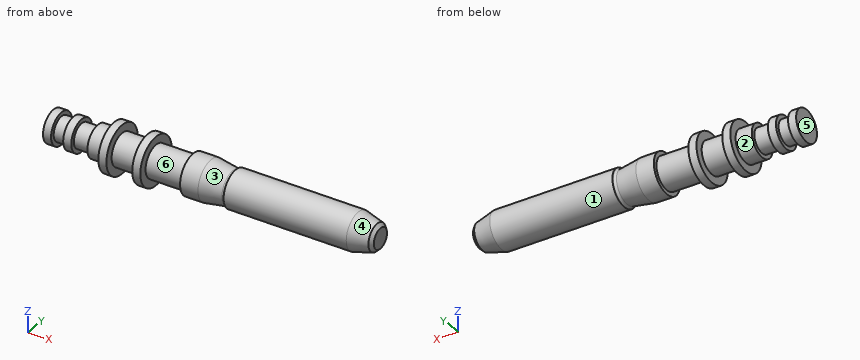
from build123d import *

# Parameters (mm, degrees)
FILLET1_R      = 0.0762
CHAMFER1_SIZE  = 0.0762
CHAMFER1_SIZE2 = 0.107763073


with BuildPart() as part:
    # Sketch1 → Revolve1 (revolve)
    with BuildSketch(Plane.XY, mode=Mode.PRIVATE) as revolve1_sk:
        Polygon((6.955835037, 0.508), (6.955835037, 0), (17.242835037, 0), (17.242835037, 0.397037489), (16.544335037, 0.5842), (12.686075037, 0.5842), (12.648252987, 0.518690288), (11.913915037, 0.635), (11.350035037, 0.635), (11.350035037, 0.508), (10.181635037, 0.508), (10.181635037, 0.762), (9.927635037, 0.762), (9.927635037, 0.508), (9.114835037, 0.508), (9.114835037, 0.762), (8.860835037, 0.762), (8.860835037, 0.508), (8.352835037, 0.508), (8.352835037, 0.381), (7.844835037, 0.381), (7.844835037, 0.508), (7.590835037, 0.508), (7.590835037, 0.381), (7.209835037, 0.381), (7.209835037, 0.508), align=None)
    revolve(revolve1_sk.sketch.rotate(Axis((-986.284560053, 0, 0), (1, 0, 0)), 180), axis=Axis((-986.284560053, 0, 0), (1, 0, 0)))

    # Fillet1
    fillet1_edges = [part.edges().sort_by_distance(p)[0] for p in [
        (12.648252987, 0.518690288, 0),
    ]]
    fillet(fillet1_edges, radius=FILLET1_R)

    # Chamfer1
    chamfer1_edges = [part.edges().sort_by_distance(p)[0] for p in [
        (17.242835037, 0.397037489, 0),
    ]]
    chamfer1_side = [part.faces().sort_by_distance(p)[0] for p in [
        (17.242835037, 0, 0),
    ]]
    chamfer(chamfer1_edges, length=CHAMFER1_SIZE, length2=CHAMFER1_SIZE2, reference=chamfer1_side[0])


solid = part.part
Work out the finished part from the listing and answer in its coordinate system (mm). Face numbers are marked on the shaded views. A direction names the side the tool comes from. Coordinates: 2 decimals unless noted, no trailing zeros. Order: outer loops, then holes, each group sorted by start corner. A loop starts at its lowest first (then second) coordinate and runs counter-clockwise, first axis right, second up. Notation, with made-up numbers: (30.25, 18.5) - (52.25, 18.5) arc R24 cw to (52.25, 57.5) - close; hole circle Ø1 at (14, 15). An arc over 180 degrees is marked (long way). Put each result on its own line as item: value. Start each with the question number.
1) Find section A-A (x = 9.75). Give the vertices of the cut face in (y, z).
2) For the marked faces 1, 2 and 3, determine the directions among +Z, -Z, +X, -X, +Y, -Y from which every point of the face is accessible in a straight line to the end or side of a thin tool.
3) Find section B-B (x = 11.5). Give the vertices of the cut face in (y, z) (3 decimals), plus the area to 3 significant figures.
4) For a pull along X with two mould halves and no side action, classify the marked faces 4, 5 and 6 as released by +X, released by -X, zero draft, split by the parting line, or undercut.
5) Find the intervals of material crossed by line 1 (X direction, y = -0.2, z = -0.7); line 2 (Y direction, x = 13.5, z = -0.05), in increasing order. Write a range as from..to.
Results list:
1. outline: circle Ø1.02 at (0, 0)
2. face 1: +X
2. face 2: -X
2. face 3: none
3. outline: circle Ø1.27 at (0, 0)
3. area: 1.27 mm^2
4. face 4: released by +X
4. face 5: released by -X
4. face 6: undercut
5. line 1: x = 8.86..9.11, 9.93..10.18
5. line 2: y = -0.58..0.58
